Autodesk Inventor part; units mm, degrees
ref_plane "YZ Plane" through (0, 0, 0) normal (1, 0, 0) x (0, 1, 0)
ref_plane "XZ Plane" through (0, 0, 0) normal (0, 1, 0) x (-1, 0, 0)
ref_plane "XY Plane" through (0, 0, 0) normal (0, 0, 1) x (1, 0, 0)
sketch "Sketch1" plane through (0, 0, 0) normal (0, 1, 0) x (-1, 0, 0)
  line L0 (0, 0) -> (16, 0)
  line L1 (16, 0) -> (16, -40)
  line L2 (16, -40) -> (0, -40)
  line L3 (0, -40) -> (0, 0)
  dimension "d0" = 16
  dimension "d1" = 40
extrude "Extrusion1" add sketch "Sketch1" along normal blind 6
sketch "Sketch2" plane through (0, 6, 0) normal (0, 1, 0) x (1, 0, 0)
  line L0 (-16, 0) -> (0, 0)
  line L1 (0, 40) -> (-16, 40)
  line L2 (-16, 0) -> (-13, 0)
  line L3 (-13, 0) -> (-13, 40)
  line L4 (-13, 40) -> (-16, 40)
  line L5 (-16, 40) -> (-16, 0)
  dimension "d4" = 3
extrude "Extrusion2" add sketch "Sketch2" along normal blind 14
sketch "Sketch3" plane through (-16, 0, -40) normal (-1, 0, 0) x (0, 0, 1)
  line L0 (0, 20) -> (40, 20)
  line L1 (40, 20) -> (0, 20)
  line L2 (0, 20) -> (0, 18)
  line L3 (0, 18) -> (40, 18)
  line L4 (40, 18) -> (40, 20)
  point P0 (40, 0)
  point P1 (0, 20)
  dimension "d7" = 40
  dimension "d8" = 2
extrude "Extrusion3" add sketch "Sketch3" along normal blind 5
fillet "Fillet1" radius 1 2 edges at (-21, 20, -20) (-21, 18, -20)
fillet "Fillet2" radius 4 1 edges at (-13, 6, -20)
fillet "Fillet3" radius 3 2 edges at (0, 6, -20) (0, 0, -20)
fillet "Fillet4" radius 3 1 edges at (-16, 0, -20)
sketch "Sketch4" plane through (0, 6, 0) normal (0, 1, 0) x (1, 0, 0)
  line L0 (-8, 0) -> (-8, 10)
  line L1 (-3, 40) -> (-13, 40)
  circle A0 centre (-8, 10) radius 3
  line L2 (-8, 40) -> (-8, 30)
  line L3 (-8, 40) -> (2, 40) construction
  circle A1 centre (-8, 30) radius 3
  point P0 (0, 0)
  dimension "d15" = 10
  dimension "d16" = 6
  dimension "d17" = 10
  dimension "d18" = 90
  dimension "d19" = 5
  dimension "d20" = 6
  dimension "d23" = 5
extrude "Extrusion4" cut sketch "Sketch4" against normal through all both and the other way through all
fillet "Fillet5" radius 2 1 edges at (-16, 18, -20)
sketch "Sketch5" plane through (-16, 3, -40) normal (-1, 0, 0) x (0, 0, 1)
  line L0 (0, 5.5) -> (5, 5.5)
  line L1 (5, 5.5) -> (5, 9)
  line L2 (5, 5.5) -> (8.5, 5.5) construction
  line L3 (5, 5.5) -> (13, 5.5)
  circle A0 centre (5, 9) radius 2
  circle A1 centre (13, 5.5) radius 2
  line L4 (40, 0) -> (0, 0)
  line L5 (0, 7) -> (0, 17)
  line L6 (0, -3) -> (40, -3)
  dimension "d25" = 5
  dimension "d28" = 3.5
  dimension "d29" = 90
  dimension "d30" = 8
  dimension "d32" = 4
  dimension "d33" = 4
  dimension "d38" = 8.5
extrude "Extrusion5" cut sketch "Sketch5" against normal through all both and the other way through all
properties part number "Cable_Guide_Support_small"
Check sheet for the modelled part. Datum: model origin and axes. Units: mm. A direction names the side the tool comes from. Round coordinates to 2 decimals unless told otherwise and drop trailing zeros. Order: outer loops, then holes, each group sorted by start corner. A loop starts at its lowest first (then second) coordinate and runs counter-clockwise, first axis right, second up. Notation, with made-up numbers: (-38.5, -17) -> (7.5, -17) arc R29 ccw to (7.5, 3) -> close; hole circle Ø11 at (85, -9). An arc over 180 degrees is marked (long way). Use CSV: the item, a comma, the result in double quotes.
(1) Cross-section at D-D (y = 1.5). Record the boundary of the cut face in (x, z), and give its area (3 significant figures).
Worked out:
outline,"(-15.6, -40) -> (-0.4, -40) -> (-0.4, 0) -> (-15.6, 0) -> close; hole circle Ø6 at (-8, -30); hole circle Ø6 at (-8, -10)"
area,"551 mm²"
(2) Tool access check on faces 5 (the face through (-0.9, 0.86, -19.72)), 6 (the face through (-6, 6, -20)), 7 (the face through (-19, 18, -20)). Record the directions out of +Z, -Z, +X, -X, +Y, -Y that give a thin tool (end or side, any length) a straight path to the whole face; none if there is none.
Worked out:
face 5,"+Z, -Z, +X, -Y"
face 6,"+Z, -Z, +X, +Y"
face 7,"+Z, -Z, -X, -Y"
(3) Depth check by flat-ended pin: pin 1 (2.5 mm diameter, centred on y = 12, z = -35, fed in from -X); pin 2 (3 mm diameter, centred on y = 16.5, z = -17.5, fed in from +X); pin 3 (5 mm diameter, centred on y = 3.5, z = -26, fed in from -X); pin 4 (10.5 mm diameter, centred on y = 12.5, z = -27, fed in from -X). Enter the tip coordinate at first touch or a pass-through.
Worked out:
pin 1,"through"
pin 2,"x = -13"
pin 3,"x = -16"
pin 4,"x = -17.03"
(4) Cross-section at B-B (y = 12). Record the boundary of the cut face in (x, z), and give its area (3 significant figures).
Worked out:
outline,"(-16, -40) -> (-13, -40) -> (-13, -37) -> (-16, -37) -> close; (-16, -33) -> (-13, -33) -> (-13, 0) -> (-16, 0) -> close"
area,"108 mm²"
(5) Material ranges on line 1 along Z through (x, y) = (-13.65, 12); line 2 along Z through (x, y) = (-8.75, 1.5); line 3 along Y through (x, z) = (-4.75, -35.5), recorded low to high. Write a range as from..to.
Worked out:
line 1,"-40..-37, -33..0"
line 2,"-40..-32.9, -27.1..-12.9, -7.1..0"
line 3,"0..6"
(6) Draft check along Y on faces 1 (the face through (-20.715, 18.301, -19.72)), 2 (the face through (-11.797, 7.141, -20.28)), 3 (the face through (-14.066, 6.548, -27.434)), 4 (the face through (-16, 9, -20)). Enter one of: pulls with the +Y half, pulls with the -Y half, needs draft (parallel to the pull), parting line crosses it, or undercut.
Worked out:
face 1,"pulls with the -Y half"
face 2,"pulls with the +Y half"
face 3,"undercut"
face 4,"needs draft"
